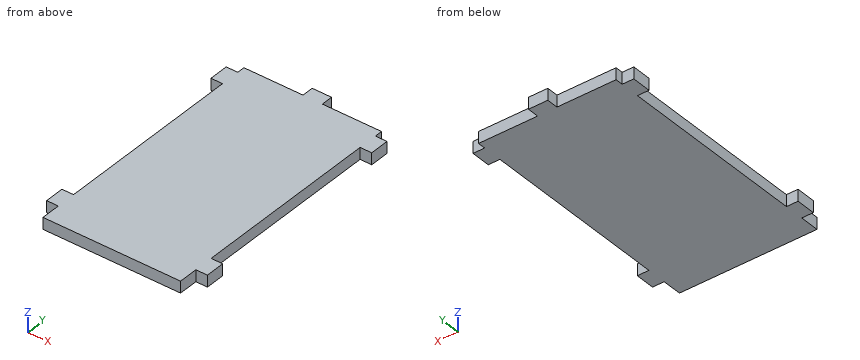
from build123d import *

# Parameters (mm, degrees)
F0_W     = 12
F0_H     = 20
F1_DEPTH = 12


# Not quite as in the source:
# - a feature names something its author has since deleted; it is built from what else it names


with BuildPart() as f1:
    # F0 (on Top) → F1 (new body)
    with BuildSketch(Plane.XY):
        with Locations((-77.025, 107.52248)):
            Rectangle(F0_W, F0_H)
        Polygon((71.025, 125.52248), (10, 125.52248), (-10, 125.52248), (-71.025, 125.52248), (-71.025, 117.52248), (-71.025, 97.52248), (-71.025, -97.52248), (-71.025, -117.52248), (-71.025, -137.52248), (71.025, -137.52248), (71.025, -117.52248), (71.025, -97.52248), (71.025, 97.52248), (71.025, 117.52248), align=None)
        with Locations((77.025, 107.52248)):
            Rectangle(F0_W, F0_H)
        with Locations((-77.025, -107.52248)):
            Rectangle(F0_W, F0_H)
        with Locations((77.025, -107.52248)):
            Rectangle(F0_W, F0_H)
        Polygon((10, 127.52248), (10, 137.52248), (-10, 137.52248), (-10, 127.52248), (-10, 125.52248), (10, 125.52248), align=None)
    extrude(amount=F1_DEPTH)


solid = f1.part
Part model, mm, in its own coordinate system. Round coordinates to 2 decimals unless told otherwise and drop trailing zeros. Write each loop counter-clockwise with the first axis right and the second up, starting at its lowest first coordinate (ties: lowest second). Pieces come first, ordered by that corner, then holes. Notation, with made-up numbers: M 39.5,88 L 85.5,88 A20 cw 85.5,116 Z; hole C -18,48.5 d5. An arc over 180 degrees is marked long. Return JSON: item names as keys, results as strings. Group by question number.
(1) Saw through at C-C on y = 75.5. Write the cut outline in (x, z) (3 decimals), then the cut area to 3 significant figures.
(2) Saw through at A-A on z = 5.5. Write the cut outline in (x, y) (3 decimals).
(3) Pin check, flat tips, straight feed: pin 1 Ø6 at (x, z) = (59.5, 6.5) entering from +Y; pin 2 Ø3.5 at (x, z) = (-74.5, 3) entering from +Y; pin 3 Ø1 at (y, z) = (85, 9.5) entering from -X (3 decimals). Stop position of each tip, or through.
(4) Drill centre lines: probe 1 along X at (y, z) = (34.5, 8.75) (3 decimals); probe 2 along Y at (x, z) = (54, 4.75). Where is each one in solid material? Low to high.
(5) Saw through at B-B on x = -44. Write the cut outline in (y, z).
Returned:
{
 "1": {"outline": "M -71.025,0 L 71.025,0 L 71.025,12 L -71.025,12 Z", "area": "1,700 mm²"},
 "2": {"outline": "M -83.025,-117.522 L -71.025,-117.522 L -71.025,-137.522 L 71.025,-137.522 L 71.025,-117.522 L 83.025,-117.522 L 83.025,-97.522 L 71.025,-97.522 L 71.025,97.522 L 83.025,97.522 L 83.025,117.522 L 71.025,117.522 L 71.025,125.522 L 10,125.522 L 10,137.522 L -10,137.522 L -10,125.522 L -71.025,125.522 L -71.025,117.522 L -83.025,117.522 L -83.025,97.522 L -71.025,97.522 L -71.025,-97.522 L -83.025,-97.522 Z"},
 "3": {"pin 1": "y = 125.52", "pin 2": "y = 117.52", "pin 3": "x = -71.025"},
 "4": {"probe 1": "-71.025 to 71.025", "probe 2": "-137.52 to 125.52"},
 "5": {"outline": "M -137.52,0 L 125.52,0 L 125.52,12 L -137.52,12 Z"}
}
